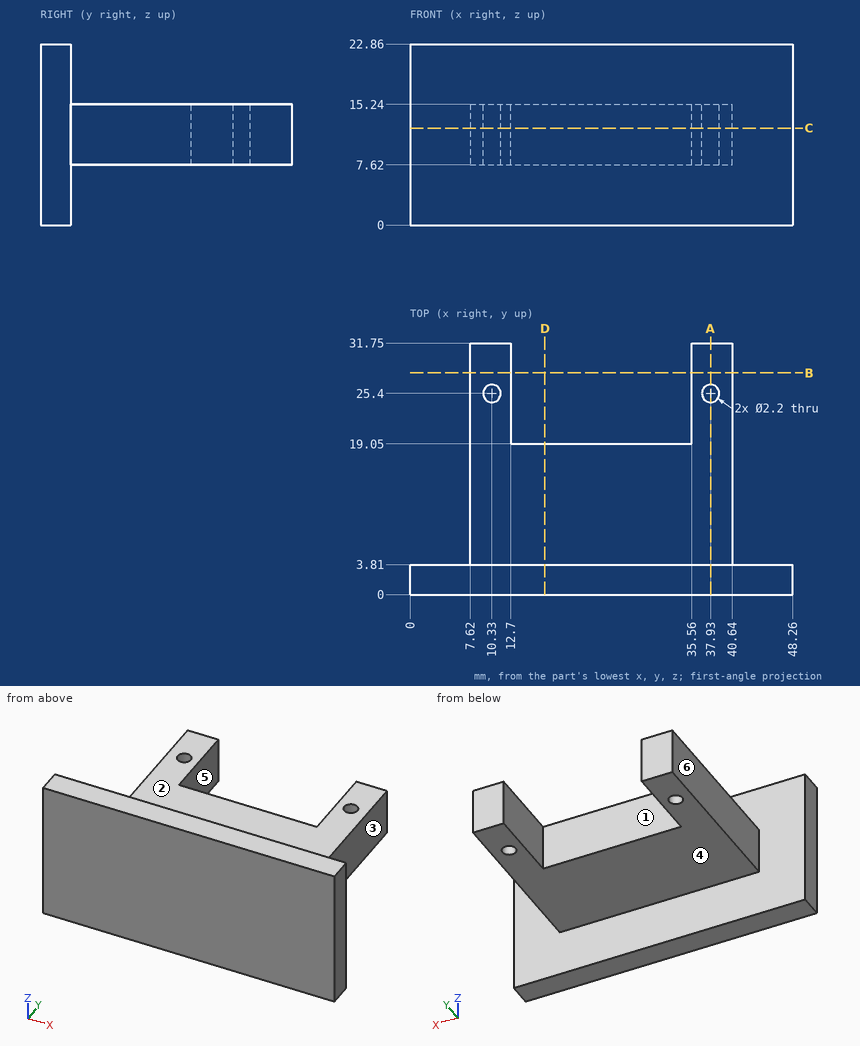
The figure shows three views and two pictorial views of one solid part (mm, origin at its lowest corner). Answer the questions. A direction names the side the tool comes from. Round coordinates to 2 decimals unless told otherwise and drop trailing zeros. Write each loop counter-clockwise with the first axis right and the second up, starting at its lowest first coordinate (ties: lowest second). Pieces come first, ordered by that corner, then holes. Notation, with made-up numbers: (-0.5, -2) -> (54.5, -2) arc R18 ccw to (54.5, 17) -> close; hole circle Ø5 at (77, 46.25). An arc over 180 degrees is marked (long way). Write each question's results on one line, items separated by ' | '.
Q1. Section D-D, the plane x = 17 is taken. Write down the section's boundary in (y, z), then the cut area to 3 significant figures.
Data:
outline: (0, 0) -> (3.81, 0) -> (3.81, 7.62) -> (19.05, 7.62) -> (19.05, 15.24) -> (3.81, 15.24) -> (3.81, 22.86) -> (0, 22.86) -> close | area: 203 mm^2
Q2. Straight lines are drawn through the part: line 1 along Y through (x, z) = (10.33, 13.5); line 2 along X through (y, z) = (26, 12.75); line 3 along Z through (x, y) = (8, 23). For each, find the intervals that lie inside material, in ascending order. Write a range as [from, to].
Data:
line 1: [0, 24.3], [26.5, 31.75] | line 2: [7.62, 9.41], [11.25, 12.7], [35.56, 37.01], [38.85, 40.64] | line 3: [7.62, 15.24]
Q3. Section A-A, the plane x = 37.93 is taken. Write down the section's boundary in (y, z), then the cut area to 3 significant figures.
Data:
outline: (0, 0) -> (3.81, 0) -> (3.81, 7.62) -> (24.3, 7.62) -> (24.3, 15.24) -> (3.81, 15.24) -> (3.81, 22.86) -> (0, 22.86) -> close; (26.5, 7.62) -> (31.75, 7.62) -> (31.75, 15.24) -> (26.5, 15.24) -> close | area: 283 mm^2
Q4. Determine the mould class of the marked faces 1, 2 and 3 for opening direction X: released by +X, released by -X, zero draft, split by the parting line, or undercut.
Data:
face 1: undercut | face 2: zero draft | face 3: released by +X
Q5. Section B-B, the plane y = 28 is taken. Write down the section's boundary in (x, z), then the cut area to 3 significant figures.
Data:
outline: (7.62, 7.62) -> (12.7, 7.62) -> (12.7, 15.24) -> (7.62, 15.24) -> close; (35.56, 7.62) -> (40.64, 7.62) -> (40.64, 15.24) -> (35.56, 15.24) -> close | area: 77.4 mm^2
Q6. Which of the six approach directions +Z, -Z, +X, -X, +Y, -Y give full straight-line access (tool end or side, diameter ignored) to the marked faces 4, 5 and 6?
Data:
face 4: -Z, +X, -X, +Y | face 5: +Z, -Z, +Y | face 6: +Z, -Z, -X, +Y
Q7. Section C-C, the plane z = 12.25 is taken. Write down the section's boundary in (x, y), then the cut area to 3 significant figures.
Data:
outline: (0, 0) -> (48.26, 0) -> (48.26, 3.81) -> (40.64, 3.81) -> (40.64, 31.75) -> (35.56, 31.75) -> (35.56, 19.05) -> (12.7, 19.05) -> (12.7, 31.75) -> (7.62, 31.75) -> (7.62, 3.81) -> (0, 3.81) -> close; hole circle Ø2.2 at (10.33, 25.4); hole circle Ø2.2 at (37.93, 25.4) | area: 809 mm^2
Q8. Flat-ended cylindrical pins translate along their axes: P1, Ø10, axis at y = 19.5, z = 13, coming from the +X side; P2, Ø8.5, axis at y = 24, z = 12, coming from the -X side; P3, Ø1.3, axis at x = 10.33, y = 25.4, coming from the +Z side; P4, Ø6, axis at x = 8.5, z = 3.5, coming from the +Y side. Find the tip coordinate at first contact, or state that the pin passes through.
Data:
P1: x = 40.64 | P2: x = 7.62 | P3: through | P4: y = 3.81
